Here's how the part is built. I have some questions about the finished solid (model axes, mm). A direction names the side the tool comes from. Round coordinates to 2 decimals unless told otherwise and drop trailing zeros. Order: outer loops, then holes, each group sorted by start corner. A loop starts at its lowest first (then second) coordinate and runs counter-clockwise, first axis right, second up. Notation, with made-up numbers: M 66.25,87.5 L 125.25,87.5 A19 ccw 125.25,116.5 Z; hole C -13.75,66 d9. An arc over 180 degrees is marked long. Write item = value, one per line. Start each with the question number.
Item 1: I want a section at B-B, the plane y = -35. List the corners of the cut face in (x, z) for me, plus the area to 3 significant figures.
Item 2: We'd pull the mould along Y, two halves only. Please class faces 4 (the face through (96.52, -58, -3)), 5 (the face through (-96.52, -32, -3)), 6 (the face through (99, -41.91, -3)), 7 (the face through (-99, -52.07, -3)): pulls with the +Y half, pulls with the -Y half, needs draft (parallel to the pull), parting line crosses it, or undercut.
Item 3: I'm going to push flat-ended pins straight in: P1, Ø2.5, axis at x = 82.5, z = -2, coming from the -Y side; P2, Ø1, axis at y = -53.5, z = -4.5, coming from the +X side; P3, Ø2.5, axis at y = -66.5, z = -2, coming from the -X side. Where does each tip first touch, or does it pass through?
Item 4: For faces 1 (the face through (-66.04, -66, -3)), 2 (the face through (0, -63.5, -3)), 3 (the face through (66.04, -66, -3)), which set-ups out of +Z, -Z, +X, -X, +Y, -Y let a thin tool reach every point of the face, with its end or its side?
Item 5: I want a section at A-A, the plane z = -2.4. List the corners of the cut face in (x, y) for me, plus the area to 3 significant figures.
Item 6: Please list where these lines run through material, in increasing order: L1, parallel to Y at x = 72, z = -2.8; L2, parallel to X at y = -33, z = -4.5.
Item 7: I want a section at C-C, the plane x = 85. List the corners of the cut face in (y, z) for me.
```python
from build123d import *

# Parameters (mm, degrees)
SKETCH1_W           = 193.04
SKETCH1_H           = 63.5
BOSS_EXTRUDE1_DEPTH = 5.08
SKETCH2_W           = 5.08
SKETCH2_H           = 10.16
BOSS_EXTRUDE2_DEPTH = 5.08
SKETCH3_W           = 30.48
SKETCH3_H           = 5.08
BOSS_EXTRUDE3_DEPTH = 5.08


with BuildPart() as part:
    # Sketch1 → Boss-Extrude1 (new body)
    with BuildSketch(Plane.XY):
        with Locations((0, -31.75)):
            Rectangle(SKETCH1_W, SKETCH1_H)
    extrude(amount=-BOSS_EXTRUDE1_DEPTH)

    # Sketch2 → Boss-Extrude2 (add)
    with BuildSketch(Plane.XY):
        with Locations((99.06, -46.99)):
            Rectangle(SKETCH2_W, SKETCH2_H)
        with Locations((99.06, -16.51)):
            Rectangle(SKETCH2_W, SKETCH2_H)
        with Locations((-99.06, -46.99)):
            Rectangle(SKETCH2_W, SKETCH2_H)
        with Locations((-99.06, -16.51)):
            Rectangle(SKETCH2_W, SKETCH2_H)
    extrude(amount=-BOSS_EXTRUDE2_DEPTH)

    # Sketch3 → Boss-Extrude3 (add)
    with BuildSketch(Plane.XZ.offset(63.5)):
        with Locations((50.8, -2.54)):
            Rectangle(SKETCH3_W, SKETCH3_H)
        with Locations((-50.8, -2.54)):
            Rectangle(SKETCH3_W, SKETCH3_H)
    extrude(amount=BOSS_EXTRUDE3_DEPTH)


solid = part.part
```
Filled in:
q1.outline = M -96.52,-5.08 L 96.52,-5.08 L 96.52,0 L -96.52,0 Z
q1.area = 981 mm^2
q2.face_4 = needs draft
q2.face_5 = undercut
q2.face_6 = undercut
q2.face_7 = pulls with the -Y half
q3.P1 = -63.5
q3.P2 = 96.52
q3.P3 = -66.04
q4.face_1 = +Z, -Z, -X, -Y
q4.face_2 = +Z, -Z, -Y
q4.face_3 = +Z, -Z, +X, -Y
q5.outline = M -101.6,-52.07 L -96.52,-52.07 L -96.52,-63.5 L -66.04,-63.5 L -66.04,-68.58 L -35.56,-68.58 L -35.56,-63.5 L 35.56,-63.5 L 35.56,-68.58 L 66.04,-68.58 L 66.04,-63.5 L 96.52,-63.5 L 96.52,-52.07 L 101.6,-52.07 L 101.6,-41.91 L 96.52,-41.91 L 96.52,-21.59 L 101.6,-21.59 L 101.6,-11.43 L 96.52,-11.43 L 96.52,0 L -96.52,0 L -96.52,-11.43 L -101.6,-11.43 L -101.6,-21.59 L -96.52,-21.59 L -96.52,-41.91 L -101.6,-41.91 Z
q5.area = 12,800 mm^2
q6.L1 = -63.5 to 0
q6.L2 = -96.52 to 96.52
q7.outline = M -63.5,-5.08 L 0,-5.08 L 0,0 L -63.5,0 Z
